For this review, take the finished solid that the model builds, in its own axes (mm). Face numbers are marked on the shaded views. A direction names the side the tool comes from. Give positions to 0.01 mm unless a question says otherwise; leave off trailing zeros. Loops run counter-clockwise (first coordinate to the right, second up) from the corner with the lowest first, then second, coordinate; pieces in that order, holes last.
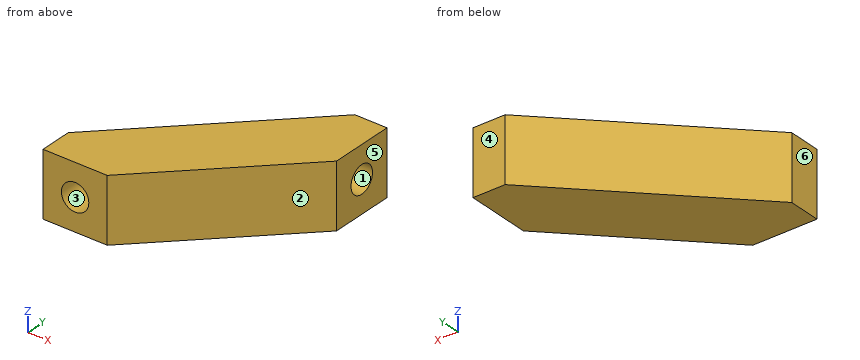
```python
from build123d import *

# Parameters (mm, degrees)
F1_DEPTH = 6.35
F2_R     = 1.35255
F3_DEPTH = 3.175
F4_R     = 1.35255
F5_DEPTH = 3.175


with BuildPart() as f1:
    # F0 (on Top) → F1 (new body)
    with BuildSketch(Plane.XY):
        Polygon((-19.05, 0), (-12.7, 0), (0, 12.7), (0, 19.05), (-3.175, 19.05), (-19.05, 3.175), align=None)
    extrude(amount=F1_DEPTH)

    # F2 (on face) → F3 (cut)
    with BuildSketch(Plane.YZ):
        with Locations((15.875, 3.175)):
            Circle(F2_R)
    extrude(amount=-F3_DEPTH, mode=Mode.SUBTRACT)

    # F4 (on face) → F5 (cut)
    with BuildSketch(Plane.XZ):
        with Locations((-15.875, 3.175)):
            Circle(F4_R)
    extrude(amount=-F5_DEPTH, mode=Mode.SUBTRACT)


solid = f1.part
```
Q1. For pin 1 Ø1.5 at (x, z) = (-13, 2) entering from +Y (3 decimals); pin 2 Ø1.6 at (x, z) = (-15.875, 3.175) entering from -Y (3 decimals); pin 3 Ø1.6 at (y, z) = (15.875, 3.175) entering from -X, all flat-tipped, find the tip position at first contact; note any pin that passes through.
Answers:
pin 1: stops at y = 9.975
pin 2: stops at y = 3.175
pin 3: stops at x = -7.15
Q2. For probe 1 along X at (y, z) = (2.75, 2); probe 2 along X at (y, z) = (10.5, 3.75) (3 decimals); probe 3 along Y at (x, z) = (-9.75, 4) (3 decimals), list the stretches that pass through material, from the lowest coordinate up.
Answers:
probe 1: x = -19.05 to -16.54, -15.21 to -9.95
probe 2: x = -11.725 to -2.2
probe 3: y = 2.95 to 12.475
Q3. Consider section A-A on x = -2.75. Give the boundary of the cut face in (y, z) (3 decimals).
Answers:
outline: (9.95, 0) - (19.05, 0) - (19.05, 6.35) - (9.95, 6.35) - close; hole circle Ø2.705 at (15.875, 3.175)
Q4. Machinability: for the marked faces 1 and 2, which of the approach directions +Z, -Z, +X, -X, +Y, -Y give a long, thin tool a straight path to every point of the face, cutting with its end or side? Answer none if there is none.
Answers:
face 1: +X
face 2: +Z, -Z, +X, -Y
Q5. Consider section B-B on y = 2. Give the boundary of the cut face in (x, z) (3 decimals).
Answers:
outline: (-19.05, 0) - (-10.7, 0) - (-10.7, 6.35) - (-19.05, 6.35) - close; hole circle Ø2.705 at (-15.875, 3.175)
Q6. Mouldability with a two-part tool opening along X and no side actions: class the marked faces 3, 4, 5 and 6 as +X half, -X half, draft (parallel to the pull), parting line (faces both ways), or undercut.
Answers:
face 3: undercut
face 4: draft
face 5: +X half
face 6: -X half
Q7. Consider section D-D on y = 15. Give the boundary of the cut face in (x, z) (3 decimals), plus the area to 3 significant figures.
Answers:
outline: (-7.225, 0) - (0, 0) - (0, 2.144) - (-3.175, 2.144) - (-3.175, 4.206) - (0, 4.206) - (0, 6.35) - (-7.225, 6.35) - close
area: 39.3 mm2
Q8. Consider section C-C on z = 5.75. Give the boundary of the cut face in (x, y) (3 decimals), plus the area to 3 significant figures.
Answers:
outline: (-19.05, 0) - (-12.7, 0) - (0, 12.7) - (0, 19.05) - (-3.175, 19.05) - (-19.05, 3.175) - close
area: 156 mm2
